Source: three-view drawing plus pictorial views. Frame: mm from the lowest corner of the part. A direction names the side the tool comes from. Give positions to 0.01 mm unless a question says otherwise; leave off trailing zeros. Loops run counter-clockwise (first coordinate to the right, second up) from the corner with the lowest first, then second, coordinate; pieces in that order, holes last. Notation, with made-up numbers: (41.5, 73.5) - (78.5, 73.5) arc R32 cw to (78.5, 101.5) - close; hole circle Ø5 at (-4.75, 76.25). An arc over 180 degrees is marked (long way). Answer as a JSON object with one key per item and string values. Group by question number.
(1) Section query B-B (y = 15.35). Return loops of the section in (x, z), plus the area to 3 significant figures.
(2) Section query A-A (x = 33.5). Return loops of the section in (y, z), plus the area to 3 significant figures.
(3) Pin query (flat end, axial travel): P1, Ø1.5, axis at x = 25, y = 15.5, coming from the -Z side; P2, Ø2.5, axis at x = 19.5, z = 4, coming from the +Y side; P3, Ø5.5, axis at x = 33.5, y = 22.85, coming from the -Z side. Return the tip coordinate at first contact, or that it passes through.
(4) Section query C-C (z = 2.25). Return loops of the section in (x, y).
(5) Material intervals for L1, parallel to Y at x = 13.5, z = 11.15; L2, parallel to X at y = 7.5, z = 8.75; L3, parallel to Y at x = 13.5, z = 7.45, sorted ascending.
(6) Section query D-D (x = 41.5). Return loops of the section in (y, z).
(7) Access query for the marked faces 1, 2 and 3. Directions: +Z, -Z, +X, -X, +Y, -Y. A direction counts if a zero-diameter tool reaches every point of the face in a straight line with its end or side. Return the directions, or none.
(8) Mould query, pull axis Y, two halves, no side actions, for the marked faces 4, 5 and 6. Classes: +Y half, -Y half, draft (parallel to the pull), parting line (faces both ways), or undercut.
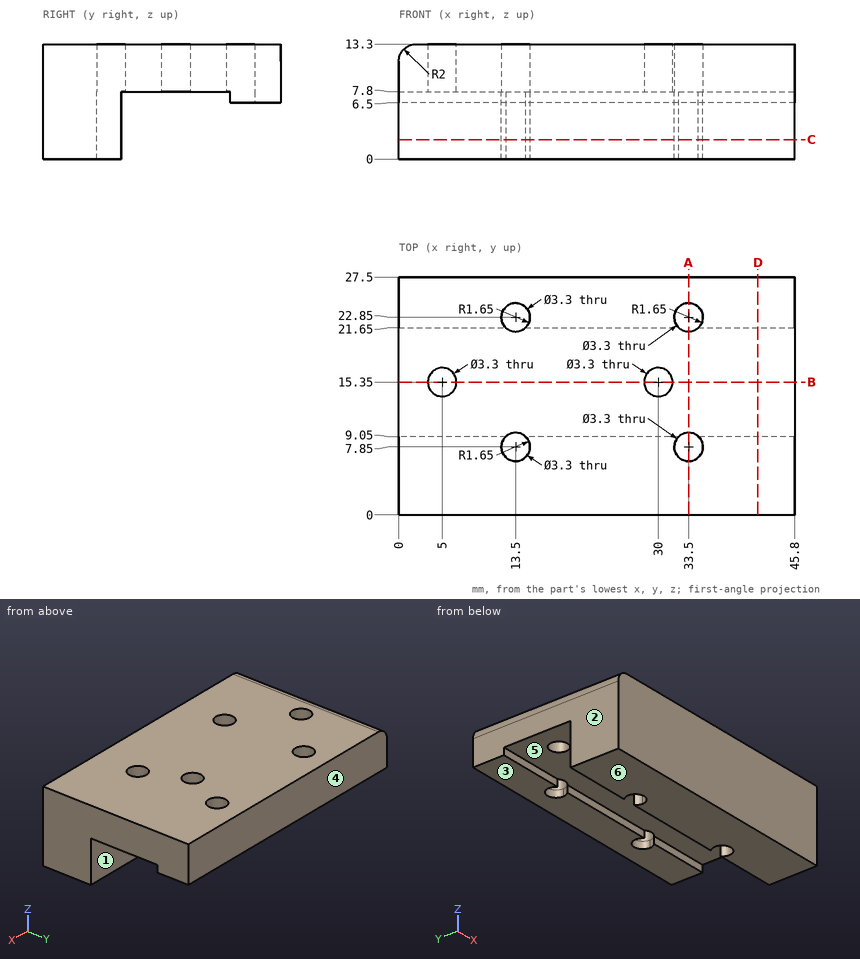
Recorded:
{
 "1": {"outline": "(0, 7.8) - (3.35, 7.8) - (3.35, 13.3) - (2, 13.3) arc R2 ccw to (0, 11.3) - close; (6.65, 7.8) - (28.35, 7.8) - (28.35, 13.3) - (6.65, 13.3) - close; (31.65, 7.8) - (45.8, 7.8) - (45.8, 13.3) - (31.65, 13.3) - close", "area": "215 mm^2"},
 "2": {"outline": "(0, 0) - (6.2, 0) - (6.2, 13.3) - (0, 13.3) - close; (9.5, 7.8) - (21.2, 7.8) - (21.2, 13.3) - (9.5, 13.3) - close; (24.5, 6.5) - (27.5, 6.5) - (27.5, 13.3) - (24.5, 13.3) - close", "area": "167 mm^2"},
 "3": {"P1": "stops at z = 7.8", "P2": "stops at y = 9.05", "P3": "stops at z = 6.5"},
 "4": {"outline": "(0, 0) - (45.8, 0) - (45.8, 9.05) - (34.63, 9.05) arc R1.65 cw (long way) to (32.37, 9.05) - (14.63, 9.05) arc R1.65 cw (long way) to (12.37, 9.05) - (0, 9.05) - close"},
 "5": {"L1": "y = 0 to 6.2, 9.5 to 21.2, 24.5 to 27.5", "L2": "x = 0 to 11.89, 15.11 to 31.89, 35.11 to 45.8", "L3": "y = 0 to 6.2, 24.5 to 27.5"},
 "6": {"outline": "(0, 0) - (9.05, 0) - (9.05, 7.8) - (21.65, 7.8) - (21.65, 6.5) - (27.5, 6.5) - (27.5, 13.3) - (0, 13.3) - close"},
 "7": {"face 1": "-Z, +X, -X", "face 2": "+Z, -Z, -X, +Y, -Y", "face 3": "-Z, +X, -X, +Y"},
 "8": {"face 4": "+Y half", "face 5": "undercut", "face 6": "draft"}
}
